Here's how the part is built. I have some questions about the finished solid (model axes, mm). Face numbers are marked on the shaded views. A direction names the side the tool comes from. Coordinates: 2 decimals unless noted, no trailing zeros. Order: outer loops, then holes, each group sorted by start corner. A loop starts at its lowest first (then second) coordinate and runs counter-clockwise, first axis right, second up. Notation, with made-up numbers: M -32.75,-29 L -16.75,-29 A9 cw -16.75,-16 Z; hole C 17.5,52 d6. An arc over 180 degrees is marked long. One line per question, with ' | ' between items. Start each with the question number.
```python
from build123d import *

# Parameters (mm, degrees)
F1_W     = 45
F1_H     = 75
F1_W_2   = 40
F1_H_2   = 70.19363
F3_DEPTH = 20
F2_W     = 75
F2_H     = 100
F2_W_2   = 45
F2_H_2   = 75
F4_DEPTH = 25


with BuildPart() as f3:
    # F1 (on face) → F3 (new body)
    with BuildSketch(Plane.XZ):
        with Locations((0, -0.096815)):
            Rectangle(F1_W, F1_H)
        Rectangle(F1_W_2, F1_H_2, mode=Mode.SUBTRACT)
    extrude(amount=F3_DEPTH)

    # F2 (on face) → F4 (join)
    with BuildSketch(Plane.XZ):
        Rectangle(F2_W, F2_H)
        with Locations((0, -0.096815)):
            Rectangle(F2_W_2, F2_H_2, mode=Mode.SUBTRACT)
    extrude(amount=F4_DEPTH)


solid = f3.part
```
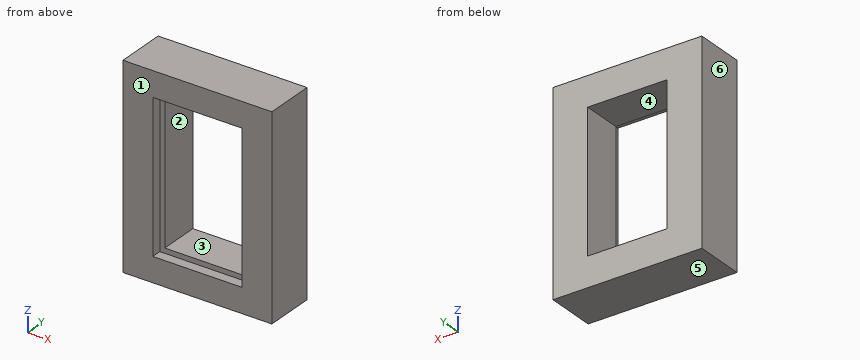
1. Imagine slicing it at A-A (z = 23). List the corners of the cut face in (x, y) for me, then the cut area to 3 significant figures.
2. Imagine slicing it at C-C (y = -5.75). List the corners of the cut face in (x, z) for me.
3. We'd pull the mould along X, two halves only. Please class the marked faces 3, 4, 5 and 6: released by +X, released by -X, zero draft, split by the parting line, or undercut.
4. Imagine slicing it at B-B (x = -9.5). List the corners of the cut face in (y, z) for me, then the cut area to 3 significant figures.
5. I need wall thicknesses on line 1 (X direction, y = -1.5, z = 6.5); line 2 (Z direction, x = -13.5, y = -13.5); line 3 (X direction, y = -20.75, z = -7). Which ranges of each line are inside material? Lowest first, please.
6. Which directions (+Z, -Z, +X, -X, +Y, -Y) give clear straight access to the entire face, cutting with the end or side of a thin tool? Please do the marked faces 1 and 2.
Entries:
1) outline: M -37.5,-25 L -22.5,-25 L -22.5,-20 L -20,-20 L -20,0 L -37.5,0 Z; M 20,-20 L 22.5,-20 L 22.5,-25 L 37.5,-25 L 37.5,0 L 20,0 Z | area: 850 mm²
2) outline: M -37.5,-50 L 37.5,-50 L 37.5,50 L -37.5,50 Z; hole M -20,-35.1 L 20,-35.1 L 20,35.1 L -20,35.1 Z
3) face 3: undercut | face 4: undercut | face 5: zero draft | face 6: released by -X
4) outline: M -25,-50 L 0,-50 L 0,-35.1 L -20,-35.1 L -20,-37.6 L -25,-37.6 Z; M -25,37.4 L -20,37.4 L -20,35.1 L 0,35.1 L 0,50 L -25,50 Z | area: 721 mm²
5) line 1: -37.5 to -20, 20 to 37.5 | line 2: -50 to -35.1, 35.1 to 50 | line 3: -37.5 to -22.5, 22.5 to 37.5
6) face 1: +Z, -Z, +X, -X, -Y | face 2: +Y, -Y
